Build history of the part. All positions in model axes, mm. Face numbers are marked on the shaded views. A direction names the side the tool comes from. Round coordinates to 2 decimals unless told otherwise and drop trailing zeros. Write each loop counter-clockwise with the first axis right and the second up, starting at its lowest first coordinate (ties: lowest second). Pieces come first, ordered by that corner, then holes.
Item 1: 3-axis set-ups, long thin cutter, end or side, ignore diameter. For the marked faces 1 and 2: which of +Z, -Z, +X, -X, +Y, -Y reach the whole face in a straight line?
Item 2: Drop flat-ended pins along their axis: pin 1 Ø2 at (y, z) = (-13, 16) entering from +X; pin 2 Ø3.5 at (x, y) = (15, -11) entering from +Z. Give the stop position or say it passes through.
Item 3: Band-saw the part on D-D, the plane y = -1.75. Write the cut outline in (x, z), then the cut area to 4 significant figures.
Item 4: Band-saw the part on B-B, the plane x = 19. Write the cut outline in (y, z).
Item 5: Mould opens along Y. For the marked faces 3, 4, 5 and 6 say: +Y half, -Y half, draft (parallel to the pull), parting line (faces both ways), or undercut.
Item 6: Wall check: probe 1 along Z at (x, y) = (3.4, -10); probe 2 along Y at (x, z) = (8.5, 5.5); probe 3 along Y at (x, z) = (1.4, 15). Give the ranges that are in metal, low to high.
Item 7: Band-saw the part on C-C, the plane z = 15. Write the cut outline in (x, y), then the cut area to 3 significant figures.
Item 8: Band-saw the part on A-A, the plane y = -10. Write the cut outline in (x, z).
```python
from build123d import *

# Parameters (mm, degrees)
F1_DEPTH = 20
F2_W     = 25.5
F2_H     = 12
F3_DEPTH = 26
F4_R     = 3.15
F5_DEPTH = 25
F6_R     = 3.15
F7_DEPTH = 25


with BuildPart() as f1:
    # F0 (on Front) → F1 (new body)
    with BuildSketch(Plane.XZ):
        Polygon((0, 30), (0, 0), (30, 0), (30, 4), (4.5, 30), align=None)
    extrude(amount=F1_DEPTH)

    # F2 (on face) → F3 (cut)
    with BuildSketch(Plane.XY.offset(30)):
        with Locations((17.25, -10)):
            Rectangle(F2_W, F2_H)
    extrude(amount=-F3_DEPTH, mode=Mode.SUBTRACT)

    # F4 (on Right) → F5 (cut)
    with BuildSketch(Plane.YZ):
        with Locations((-10, 15)):
            Circle(F4_R)
    extrude(amount=F5_DEPTH, mode=Mode.SUBTRACT)

    # F6 (on face) → F7 (cut)
    with BuildSketch(Plane.XY.offset(4)):
        with Locations((18, -10)):
            Circle(F6_R)
    extrude(amount=-F7_DEPTH, mode=Mode.SUBTRACT)


solid = f1.part
```
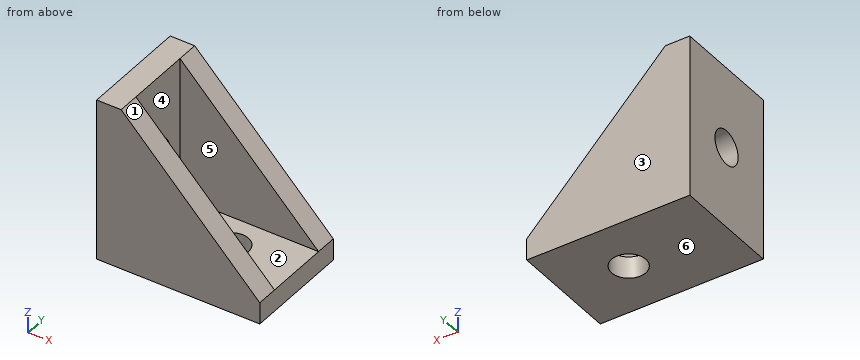
Results:
1. face 1: +Z, +X, +Y, -Y
1. face 2: +Z, +X
2. pin 1: stops at x = 4.5
2. pin 2: stops at z = 4
3. outline: (0, 0) - (30, 0) - (30, 4) - (4.5, 30) - (0, 30) - close
3. area: 568.5 mm2
4. outline: (-20, 0) - (-12.99, 0) - (-12.99, 4) - (-16, 4) - (-16, 15.22) - (-20, 15.22) - close; (-7.01, 0) - (0, 0) - (0, 15.22) - (-4, 15.22) - (-4, 4) - (-7.01, 4) - close
5. face 3: +Y half
5. face 4: undercut
5. face 5: undercut
5. face 6: draft
6. probe 1: z = 0 to 11.85, 18.15 to 30
6. probe 2: y = -20 to -16, -4 to 0
6. probe 3: y = -20 to -13.15, -6.85 to 0
7. outline: (0, -20) - (19.21, -20) - (19.21, -16) - (4.5, -16) - (4.5, -13.15) - (0, -13.15) - close; (0, -6.85) - (4.5, -6.85) - (4.5, -4) - (19.21, -4) - (19.21, 0) - (0, 0) - close
7. area: 179 mm2
8. outline: (0, 0) - (14.85, 0) - (14.85, 4) - (4.5, 4) - (4.5, 11.85) - (0, 11.85) - close; (0, 18.15) - (4.5, 18.15) - (4.5, 30) - (0, 30) - close; (21.15, 0) - (30, 0) - (30, 4) - (21.15, 4) - close
